Answer from the drawing. Dimensions are ordinates in mm from the lowest x, y and z of the part. Give positions to 0.01 mm unless a question says otherwise; leave off trailing zeros. Write each loop counter-clockwise with the first axis right and the second up, starting at its lowest first coordinate (ties: lowest second). Pieces come first, ordered by that corner, then holes. Notation, with made-up numbers: M 59,88 L 112,88 A24 ccw 112,124 Z; hole C -32.5,-7 d6. An arc over 180 degrees is marked long. Put each result on its own line as item: value.
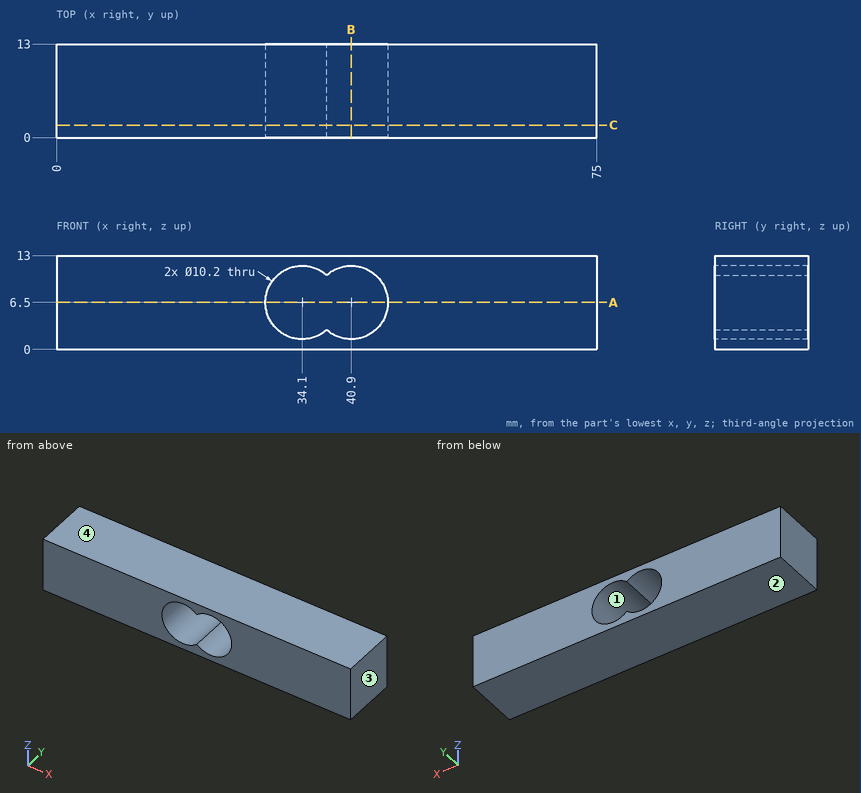
(1) Section A-A on z = 6.5 is taken. Determine the outline of the cut face in (x, y), and give its area (3 significant figures).
Result:
outline: M 0,0 L 29,0 L 29,13 L 0,13 Z; M 46,0 L 75,0 L 75,13 L 46,13 Z
area: 754 mm²
(2) Section B-B on x = 40.9 is taken. Determine the outline of the cut face in (y, z), and give its area (3 significant figures).
Result:
outline: M 0,0 L 13,0 L 13,1.4 L 0,1.4 Z; M 0,11.6 L 13,11.6 L 13,13 L 0,13 Z
area: 36.4 mm²
(3) Straight lines are drawn through the part: line 1 along Z through (x, y) = (34.1, 5); line 2 along X through (y, z) = (10, 6.75); line 3 along Z through (x, y) = (45, 2.75). For each, find the intervals that lie inside material, in ascending order. Write a range as from..to.
Result:
line 1: z = 0..1.4, 11.6..13
line 2: x = 0..29.01, 45.99..75
line 3: z = 0..3.47, 9.53..13
(4) Section C-C on y = 1.75 is taken. Determine the outline of the cut face in (x, z).
Result:
outline: M 0,0 L 75,0 L 75,13 L 0,13 Z; hole M 37.5,2.7 A5.1 ccw long 37.5,10.3 A5.1 ccw long Z
(5) For a pull along Z with two mould halves and no side action, classify the marked faces 1, 2, 3 and 4 as +Z half, -Z half, draft (parallel to the pull), parting line (faces both ways), or undercut.
Result:
face 1: undercut
face 2: -Z half
face 3: draft
face 4: +Z half
